Verification items for the finished model (mm, model axes). A direction names the side the tool comes from. Round coordinates to 2 decimals unless told otherwise and drop trailing zeros. Write each loop counter-clockwise with the first axis right and the second up, starting at its lowest first coordinate (ties: lowest second). Pieces come first, ordered by that corner, then holes. Notation, with made-up numbers: M 61,-31.75 L 106,-31.75 A26 ccw 106,-13.75 Z; hole C 19.5,77.5 d7. An arc over 180 degrees is marked long. One line per question, with ' | ' between items.
from build123d import *

# Parameters (mm, degrees)
BASE_FLANGE1_DEPTH = 76.2
CUT_EXTRUDE1_DEPTH = 142.314253085
SKETCH7_R          = 3.3782
CUT_EXTRUDE2_DEPTH = 142.314253085
FILLET1_R          = 3.175


# Sheet-metal steps are written as plain solids
with BuildPart() as part:
    # Sketch1 → Base-Flange1 (new body)
    with BuildSketch(Plane.XY):
        with BuildLine():
            Line((117.475, 19.05), (117.475, 6.35))
            ThreePointArc((117.475, 6.35), (115.615128061, 1.859871939), (111.125, 0))
            Line((111.125, 0), (6.35, 0))
            ThreePointArc((6.35, 0), (1.859871939, 1.859871939), (0, 6.35))
            Line((0, 6.35), (0, 19.05))
            Line((0, 19.05), (3.175, 19.05))
            Line((3.175, 19.05), (3.175, 6.35))
            ThreePointArc((3.175, 6.35), (4.10493597, 4.10493597), (6.35, 3.175))
            Line((6.35, 3.175), (111.125, 3.175))
            ThreePointArc((111.125, 3.175), (113.37006403, 4.10493597), (114.3, 6.35))
            Line((114.3, 6.35), (114.3, 19.05))
            Line((114.3, 19.05), (117.475, 19.05))
        make_face()
    extrude(amount=BASE_FLANGE1_DEPTH)

    # Sketch6 → Cut-Extrude1 (cut, through all)
    with BuildSketch(Plane.ZY):
        with BuildLine():
            Line((35.6108, 11.1125), (35.6108, 14.2875))
            ThreePointArc((35.6108, 14.2875), (38.1, 16.7767), (40.5892, 14.2875))
            Line((40.5892, 14.2875), (40.5892, 11.1125))
            ThreePointArc((40.5892, 11.1125), (38.1, 8.6233), (35.6108, 11.1125))
        make_face()
        with BuildLine():
            Line((10.2108, 11.1125), (10.2108, 14.2875))
            ThreePointArc((10.2108, 14.2875), (12.7, 16.7767), (15.1892, 14.2875))
            Line((15.1892, 14.2875), (15.1892, 11.1125))
            ThreePointArc((15.1892, 11.1125), (12.7, 8.6233), (10.2108, 11.1125))
        make_face()
        with BuildLine():
            Line((61.0108, 11.1125), (61.0108, 14.2875))
            ThreePointArc((61.0108, 14.2875), (63.5, 16.7767), (65.9892, 14.2875))
            Line((65.9892, 14.2875), (65.9892, 11.1125))
            ThreePointArc((65.9892, 11.1125), (63.5, 8.6233), (61.0108, 11.1125))
        make_face()
    extrude(amount=-CUT_EXTRUDE1_DEPTH, mode=Mode.SUBTRACT)

    # Sketch7 → Cut-Extrude2 (cut, through all)
    with BuildSketch(Plane.XZ):
        with Locations(Location((92.075, 38.1, 0), (0, 0, 270))):
            Circle(SKETCH7_R)
        with Locations(Location((25.4, 38.1, 0), (0, 0, 270))):
            Circle(SKETCH7_R)
    extrude(amount=-CUT_EXTRUDE2_DEPTH, mode=Mode.SUBTRACT)

    # Fillet1
    fillet1_edges = [part.edges().sort_by_distance(p)[0] for p in [
        (1.5875, 19.05, 0),
        (115.8875, 19.05, 0),
        (1.5875, 19.05, 76.2),
        (115.8875, 19.05, 76.2),
    ]]
    fillet(fillet1_edges, radius=FILLET1_R)


solid = part.part
1. Tool access check on faces 5 (the face through (2, 19.05, 38)), 6 (the face through (2, 13, 65.989)), 7 (the face through (3.175, 17, 38)). Record the directions out of +Z, -Z, +X, -X, +Y, -Y that give a thin tool (end or side, any length) a straight path to the whole face; none if there is none.
Results:
face 5: +Z, -Z, +X, -X, +Y | face 6: +X, -X | face 7: +Z, -Z, +Y
2. Mould release check, pull along Z, two halves, no side actions. Record for faces 1 (the face through (59, 2, 0)), 2 (the face through (113.345, 4.08, 37.567)), 3 (the face through (115.865, 16.776, 63.445)), 4 (the face through (1.61, 18.1, 75.29)): pulls with the +Z half, pulls with the -Z half, needs draft (parallel to the pull), parting line crosses it, or undercut.
Results:
face 1: pulls with the -Z half | face 2: needs draft | face 3: undercut | face 4: pulls with the +Z half
3. Go/stop test with flat-tipped pins: P1, Ø10, axis at y = 5.5, z = 67.5, coming from the +X side (3 decimals); P2, Ø6, axis at x = 43.5, z = 48.5, coming from the +Y side (3 decimals). Record where each tip stops, or that it passes through.
Results:
P1: stops at x = 117.475 | P2: stops at y = 3.175
4. Section check C-C, the plane x = 25.4. Record the cut outline in (y, z) (3 decimals), then the cut area to 3 significant figures.
Results:
outline: M 0,0 L 3.175,0 L 3.175,34.722 L 0,34.722 Z; M 0,41.478 L 3.175,41.478 L 3.175,76.2 L 0,76.2 Z | area: 220 mm2
5. Thickness scan on line 1 (X direction, y = 2.1, z = 38.1); line 2 (X direction, y = 15.5, z = 30) (3 decimals); line 3 (X direction, y = 0.95, z = 38.1). Record the ranges inside material, lowest first.
Results:
line 1: x = 1.63 to 22.02, 28.78 to 88.7, 95.45 to 115.84 | line 2: x = 0 to 3.175, 114.3 to 117.475 | line 3: x = 3.01 to 22.02, 28.78 to 88.7, 95.45 to 114.47
6. Section check B-B, the plane z = 38.1. Record the cut outline in (x, y) (3 decimals).
Results:
outline: M 0,6.35 A6.35 ccw 6.35,0 L 22.022,0 L 22.022,3.175 L 6.35,3.175 A3.175 cw 3.175,6.35 L 3.175,8.623 L 0,8.623 Z; M 0,16.777 L 3.175,16.777 L 3.175,19.05 L 0,19.05 Z; M 28.778,0 L 88.697,0 L 88.697,3.175 L 28.778,3.175 Z; M 95.453,0 L 111.125,0 A6.35 ccw 117.475,6.35 L 117.475,8.623 L 114.3,8.623 L 114.3,6.35 A3.175 cw 111.125,3.175 L 95.453,3.175 Z; M 114.3,16.777 L 117.475,16.777 L 117.475,19.05 L 114.3,19.05 Z
7. Section check D-D, the plane z = 47. Record the cut outline in (x, y) (3 decimals), then the cut area to 3 significant figures.
Results:
outline: M 0,6.35 A6.35 ccw 6.35,0 L 111.125,0 A6.35 ccw 117.475,6.35 L 117.475,19.05 L 114.3,19.05 L 114.3,6.35 A3.175 cw 111.125,3.175 L 6.35,3.175 A3.175 cw 3.175,6.35 L 3.175,19.05 L 0,19.05 Z | area: 461 mm2
8. Section check A-A, the plane z = 63.5. Record the cut outline in (x, y) (3 decimals), then the cut area to 3 significant figures.
Results:
outline: M 0,6.35 A6.35 ccw 6.35,0 L 111.125,0 A6.35 ccw 117.475,6.35 L 117.475,8.623 L 114.3,8.623 L 114.3,6.35 A3.175 cw 111.125,3.175 L 6.35,3.175 A3.175 cw 3.175,6.35 L 3.175,8.623 L 0,8.623 Z; M 0,16.777 L 3.175,16.777 L 3.175,19.05 L 0,19.05 Z; M 114.3,16.777 L 117.475,16.777 L 117.475,19.05 L 114.3,19.05 Z | area: 409 mm2
